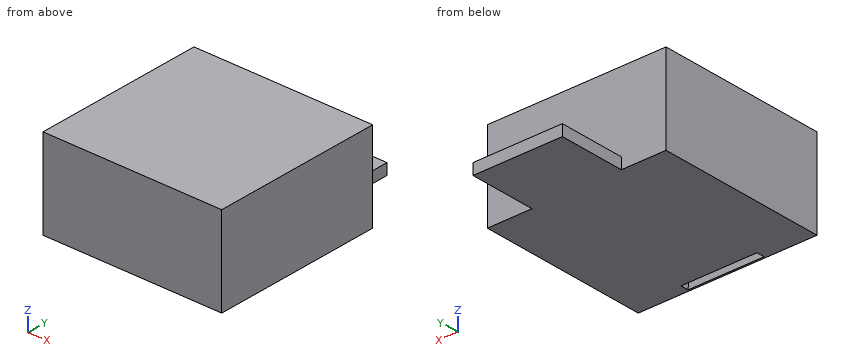
Autodesk Inventor part; units mm, degrees
ref_plane "YZ Plane" through (0, 0, 0) normal (1, 0, 0) x (0, 1, 0)
ref_plane "XZ Plane" through (0, 0, 0) normal (0, 1, 0) x (-1, 0, 0)
ref_plane "XY Plane" through (0, 0, 0) normal (0, 0, 1) x (1, 0, 0)
sketch "Sketch1" plane through (0, 0, 0) normal (0, 1, 0) x (-1, 0, 0)
  line L0 (25.4, 0) -> (-25.4, 0)
  line L1 (-25.4, 0) -> (-25.4, 25.4)
  line L2 (-25.4, 25.4) -> (25.4, 25.4)
  line L3 (25.4, 25.4) -> (25.4, 0)
  point P0 (0, 0)
  dimension "d0" = 50.8
  dimension "d1" = 25.4
extrude "Extrusion1" add sketch "Sketch1" along normal blind 2.794
sketch "Sketch2" plane through (0, 2.794, 0) normal (0, 1, 0) x (1, 0, 0)
  circle A0 centre (0, 0) radius 10.795
  dimension "d4" = 21.59
extrude "Extrusion2" cut sketch "Sketch2" against normal blind 2.286
sketch "Sketch3" plane through (0, 2.794, 0) normal (0, 1, 0) x (1, 0, 0)
  line L0 (-25.4, -25.4) -> (25.4, -25.4)
  line L1 (-25.4, -25.4) -> (25.4, -25.4)
  line L2 (25.4, -25.4) -> (25.4, 0)
  line L3 (25.4, 0) -> (-25.4, 0)
  line L4 (-25.4, 0) -> (-25.4, -25.4)
  point P0 (0, 0)
extrude "Extrusion3" add sketch "Sketch3" along normal blind 45.974
sketch "Sketch4" plane through (0, 48.768, 0) normal (0, 1, 0) x (1, 0, 0)
  line L0 (12.7, -3.175) -> (-12.7, -3.175)
  line L1 (-12.7, -3.175) -> (-12.7, 0)
  line L2 (-12.7, 0) -> (12.7, 0)
  line L3 (12.7, 0) -> (12.7, -3.175)
  point P0 (0, 0)
  dimension "d9" = 25.4
  dimension "d10" = 3.175
extrude "Extrusion4" add sketch "Sketch4" along normal blind 19.05
properties part number "half a block for magnet"
Geometry check sheet. Reference: the model listing, model coordinates, mm. Round coordinates to 2 decimals unless told otherwise and drop trailing zeros. Loops run counter-clockwise (first coordinate to the right, second up) from the corner with the lowest first, then second, coordinate; pieces in that order, holes last. Notation, with made-up numbers: (21, 84) -> (27, 84) arc R17 cw to (27, 99) -> close; hole circle Ø8 at (-8.75, -3). An arc over 180 degrees is marked (long way). Use a Markdown table: item, result.
(1) Go/stop test with flat-tipped pins: P1, Ø1.6, axis at y = 62.5, z = 1, coming from the +X side; P2, Ø5, axis at x = 16, z = 12, coming from the -Y side; P3, Ø6, axis at y = 52.5, z = 18.5, coming from the +X side; P4, Ø3, axis at x = 1, z = 7.5, coming from the +Y side. Record where each tip stops, or that it passes through.
Calculated:
| item | result |
|---|---|
| P1 | x = 12.7 |
| P2 | y = 0 |
| P3 | through |
| P4 | y = 48.77 |
(2) Sectioned sample at C-C (y = 63). Enter the section's corners in (x, z) (3 decimals), then the cut area to 3 significant figures.
Calculated:
| item | result |
|---|---|
| outline | (-12.7, 0) -> (12.7, 0) -> (12.7, 3.175) -> (-12.7, 3.175) -> close |
| area | 80.6 mm² |
(3) Scan lines: probe 1 along Y at (x, z) = (7, 22.75); probe 2 along Z at (x, y) = (12, 59) (3 decimals). Record each from-to range of solid material in increasing order.
Calculated:
| item | result |
|---|---|
| probe 1 | 0 to 48.77 |
| probe 2 | 0 to 3.175 |
(4) Sectioned sample at A-A (x = 0). Enter the section's corners in (y, z) (3 decimals).
Calculated:
| item | result |
|---|---|
| outline | (0, 0) -> (0.508, 0) -> (0.508, 10.795) -> (2.794, 10.795) -> (2.794, 0) -> (67.818, 0) -> (67.818, 3.175) -> (48.768, 3.175) -> (48.768, 25.4) -> (0, 25.4) -> close |
(5) Sectioned sample at B-B (z = 18). Enter the section's corners in (x, y).
Calculated:
| item | result |
|---|---|
| outline | (-25.4, 0) -> (25.4, 0) -> (25.4, 48.77) -> (-25.4, 48.77) -> close |
